Source: CAD feature listing. Evaluate the final solid. Frame: model axes, mm. A direction names the side the tool comes from. Round coordinates to 2 decimals unless told otherwise and drop trailing zeros. Order: outer loops, then holes, each group sorted by start corner. A loop starts at its lowest first (then second) coordinate and runs counter-clockwise, first axis right, second up. Notation, with made-up numbers: (47.5, 72.5) - (103.5, 72.5) arc R28 cw to (103.5, 91.5) - close; hole circle Ø6 at (17.25, 21). An arc over 180 degrees is marked (long way). Return JSON: item names as keys, results as strings. Group by question number.
1) Section A-A, the plane y = -49. Return loops of the section in (x, z).
2) Access query for faces 4 (the conical face through (103.076, -149.812, 9.872)), 5 (the cylindrical face through (-51.524, 147.436, 4.437)), 6 (the cylindrical face through (-113.24, -66.68, 9.26)), 7 (the cylindrical face through (1.3, 155.49, 13.14)), 8 (the cylindrical face through (-56.99, -77.15, 9.86)). Directions: +Z, -Z, +X, -X, +Y, -Y. A direction counts if a zero-diameter tool reaches every point of the face in a straight line with its end or side. Return the directions, or none.
3) Mould query, pull axis X, two halves, no side actions, for faces 1 (the conical face through (-107.812, -70.585, 9.923)), 2 (the flat face through (117.5, -2, 5)), 3 (the conical face through (-101.924, 149.812, 9.872)). Classes: pulls with the +X half, pulls with the -X half, needs draft (parallel to the pull), parting line crosses it, or undercut.
4) Contact query for flat-ended pins moving along their axis: P1, Ø6, axis at y = 145, z = 10, coming from the +X side; P2, Ø5.5, axis at y = -70, z = 10, coming from the -X side; P3, Ø6.5, axis at x = 52.5, y = -140, coming from the -Z side; P4, Ø18, axis at x = -97.5, y = 140, coming from the -Z side. Output: stop coordinate, or through.
5) Ray query, line 1 (Y direction, x = 0, z = 3.5); line 2 (X direction, y = 156, z = 10); line 3 (Y direction, x = -25.5, z = 14.5). Return the intervals inside material, ascending. Write a range as from..to.
```python
from build123d import *

# Parameters (mm, degrees)
SKETCH1_W                                            = 235
SKETCH1_H                                            = 320
BOSS_EXTRUDE1_DEPTH                                  = 20
SKETCH2_W                                            = 120
SKETCH2_H                                            = 160
CUT_EXTRUDE1_DEPTH                                   = 200.515037027
FILLET1_R                                            = 10
M3_TAPPED_HOLE1_D                                    = 2.5
M3_TAPPED_HOLE1_DEPTH                                = 10
M3_TAPPED_HOLE1_CSINK_D                              = 3.05
M3_TAPPED_HOLE1_CSINK_ANGLE                          = 90
M3_TAPPED_HOLE1_TIP                                  = 0.751075774
M3_TAPPED_HOLE2_D                                    = 2.5
M3_TAPPED_HOLE2_DEPTH                                = 8
M3_TAPPED_HOLE2_CSINK_D                              = 3.05
M3_TAPPED_HOLE2_CSINK_ANGLE                          = 90
M3_TAPPED_HOLE2_TIP                                  = 0.751075774
CBORE_FOR_M8_HEXAGON_SOCKET_HEAD_CAP_SCR_D           = 8.4
CBORE_FOR_M8_HEXAGON_SOCKET_HEAD_CAP_SCR_CBORE_D     = 15
CBORE_FOR_M8_HEXAGON_SOCKET_HEAD_CAP_SCR_CBORE_DEPTH = 9
CBORE_FOR_M12_HEXAGON_SOCKET_HEAD_CAP_SC_D           = 13
CBORE_FOR_M12_HEXAGON_SOCKET_HEAD_CAP_SC_CBORE_D     = 20
CBORE_FOR_M12_HEXAGON_SOCKET_HEAD_CAP_SC_CBORE_DEPTH = 13
M8_TAPPED_HOLE1_AT_2_COUNT                           = 2
M8_TAPPED_HOLE1_AT_2_PITCH                           = 102.5
M8_TAPPED_HOLE1_AT_3_COUNT                           = 2
M8_TAPPED_HOLE1_AT_3_PITCH                           = 205
M8_TAPPED_HOLE1_AT_4_COUNT                           = 2
M8_TAPPED_HOLE1_AT_4_PITCH                           = 50
M8_TAPPED_HOLE1_AT_5_COUNT                           = 2
M8_TAPPED_HOLE1_AT_5_PITCH                           = 155
CHAMFER1_SIZE                                        = 2
M8_TAPPED_HOLE2_AT_2_COUNT                           = 2
M8_TAPPED_HOLE2_AT_2_PITCH                           = 59.289517351
M8_TAPPED_HOLE2_AT_3_COUNT                           = 2
M8_TAPPED_HOLE2_AT_3_PITCH                           = 145
M8_TAPPED_HOLE2_AT_4_COUNT                           = 2
M8_TAPPED_HOLE2_AT_4_PITCH                           = 215
M8_TAPPED_HOLE2_AT_5_COUNT                           = 2
M8_TAPPED_HOLE2_AT_5_PITCH                           = 290


with BuildPart() as part:
    # Sketch1 → Boss-Extrude1 (new body)
    with BuildSketch(Plane.XY):
        Rectangle(SKETCH1_W, SKETCH1_H)
    extrude(amount=BOSS_EXTRUDE1_DEPTH)

    # Sketch2 → Cut-Extrude1 (cut, through all)
    with BuildSketch(Plane.XY.offset(20)):
        Rectangle(SKETCH2_W, SKETCH2_H)
    extrude(amount=-CUT_EXTRUDE1_DEPTH, mode=Mode.SUBTRACT)

    # Fillet1
    fillet1_edges = [part.edges().sort_by_distance(p)[0] for p in [
        (60, 80, 10),
        (60, -80, 10),
        (-60, -80, 10),
        (-60, 80, 10),
    ]]
    fillet(fillet1_edges, radius=FILLET1_R)

    # M3 Tapped Hole1
    with Locations(Plane(origin=(0, 0, 0), x_dir=(-1, 0, 0), z_dir=(0, 0, -1))):
        with Locations((-95, 65), (-105, 0), (-95, -65), (-65, 145), (0, 155), (65, 145)):
            CounterSinkHole(M3_TAPPED_HOLE1_D / 2, M3_TAPPED_HOLE1_CSINK_D / 2, depth=M3_TAPPED_HOLE1_DEPTH, counter_sink_angle=M3_TAPPED_HOLE1_CSINK_ANGLE)
            with Locations((0, 0, -(M3_TAPPED_HOLE1_DEPTH + M3_TAPPED_HOLE1_TIP / 2))):  # 118° drill point
                Cone(0, M3_TAPPED_HOLE1_D / 2, M3_TAPPED_HOLE1_TIP, mode=Mode.SUBTRACT)

    # M3 Tapped Hole2
    with Locations(Plane(origin=(0, 0, 0), x_dir=(-1, 0, 0), z_dir=(0, 0, -1))):
        with Locations((110, -105), (80, -140), (65, -140), (110, -120)):
            CounterSinkHole(M3_TAPPED_HOLE2_D / 2, M3_TAPPED_HOLE2_CSINK_D / 2, depth=M3_TAPPED_HOLE2_DEPTH, counter_sink_angle=M3_TAPPED_HOLE2_CSINK_ANGLE)
            with Locations((0, 0, -(M3_TAPPED_HOLE2_DEPTH + M3_TAPPED_HOLE2_TIP / 2))):  # 118° drill point
                Cone(0, M3_TAPPED_HOLE2_D / 2, M3_TAPPED_HOLE2_TIP, mode=Mode.SUBTRACT)

    # CBORE for M8 Hexagon socket head cap screws1 (through all)
    with Locations(Plane(origin=(0, 0, 0), x_dir=(-1, 0, 0), z_dir=(0, 0, -1))):
        with Locations((-52.5, 140), (-97.5, 95), (52.5, 140), (97.5, 95), (-97.5, -95), (-52.5, -140), (52.5, -140), (97.5, -95)):
            CounterBoreHole(CBORE_FOR_M8_HEXAGON_SOCKET_HEAD_CAP_SCR_D / 2, CBORE_FOR_M8_HEXAGON_SOCKET_HEAD_CAP_SCR_CBORE_D / 2, CBORE_FOR_M8_HEXAGON_SOCKET_HEAD_CAP_SCR_CBORE_DEPTH)

    # CBORE for M12 Hexagon socket head cap screws2 (through all)
    with Locations(Plane(origin=(0, 0, 0), x_dir=(-1, 0, 0), z_dir=(0, 0, -1))):
        with Locations((-97.5, 140), (97.5, 140), (-97.5, -140), (97.5, -140)):
            CounterBoreHole(CBORE_FOR_M12_HEXAGON_SOCKET_HEAD_CAP_SC_D / 2, CBORE_FOR_M12_HEXAGON_SOCKET_HEAD_CAP_SC_CBORE_D / 2, CBORE_FOR_M12_HEXAGON_SOCKET_HEAD_CAP_SC_CBORE_DEPTH)

    # Sketch24 → M8 Tapped Hole1 (revolve, cut)
    with BuildSketch(Plane(origin=(-102.5, 160, 10), x_dir=(0, 0, 1), z_dir=(1, 0, 0))):
        Polygon((0, 0), (0, 10.542926105), (3.4, 8.5), (3.4, 0.625), (4.025, 0), align=None)
    m8_tapped_hole1 = revolve(axis=Axis((-102.5, 166.35, 10), (0, -1, 0)), mode=Mode.SUBTRACT)

    # M8 Tapped Hole1 at 2: M8 Tapped Hole1 ×2
    with Locations(*[(i * M8_TAPPED_HOLE1_AT_2_PITCH, 0, 0) for i in range(1, M8_TAPPED_HOLE1_AT_2_COUNT)]):
        add(m8_tapped_hole1, mode=Mode.SUBTRACT)

    # M8 Tapped Hole1 at 3: M8 Tapped Hole1 ×2
    with Locations(*[(i * M8_TAPPED_HOLE1_AT_3_PITCH, 0, 0) for i in range(1, M8_TAPPED_HOLE1_AT_3_COUNT)]):
        add(m8_tapped_hole1, mode=Mode.SUBTRACT)

    # M8 Tapped Hole1 at 4: M8 Tapped Hole1 ×2
    with Locations(*[(i * M8_TAPPED_HOLE1_AT_4_PITCH, 0, 0) for i in range(1, M8_TAPPED_HOLE1_AT_4_COUNT)]):
        add(m8_tapped_hole1, mode=Mode.SUBTRACT)

    # M8 Tapped Hole1 at 5: M8 Tapped Hole1 ×2
    with Locations(*[(i * M8_TAPPED_HOLE1_AT_5_PITCH, 0, 0) for i in range(1, M8_TAPPED_HOLE1_AT_5_COUNT)]):
        add(m8_tapped_hole1, mode=Mode.SUBTRACT)

    # Mirror1: M8 Tapped Hole1 across plane
    add(m8_tapped_hole1.mirror(Plane.ZX), mode=Mode.SUBTRACT)

    # Mirror1 copy 1 sketch → Mirror1 copy 1 (revolve, cut)
    with BuildSketch(Plane(origin=(0, -160, 10), x_dir=(0, 0, 1), z_dir=(1, 0, 0))):
        Polygon((0, 0), (0, -10.542926105), (3.4, -8.5), (3.4, -0.625), (4.025, 0), align=None)
    revolve(axis=Axis((0, -166.35, 10), (0, -1, 0)), mode=Mode.SUBTRACT)

    # Mirror1 copy 2 sketch → Mirror1 copy 2 (revolve, cut)
    with BuildSketch(Plane(origin=(102.5, -160, 10), x_dir=(0, 0, 1), z_dir=(1, 0, 0))):
        Polygon((0, 0), (0, -10.542926105), (3.4, -8.5), (3.4, -0.625), (4.025, 0), align=None)
    revolve(axis=Axis((102.5, -166.35, 10), (0, -1, 0)), mode=Mode.SUBTRACT)

    # Mirror1 copy 3 sketch → Mirror1 copy 3 (revolve, cut)
    with BuildSketch(Plane(origin=(-52.5, -160, 10), x_dir=(0, 0, 1), z_dir=(1, 0, 0))):
        Polygon((0, 0), (0, -10.542926105), (3.4, -8.5), (3.4, -0.625), (4.025, 0), align=None)
    revolve(axis=Axis((-52.5, -166.35, 10), (0, -1, 0)), mode=Mode.SUBTRACT)

    # Mirror1 copy 4 sketch → Mirror1 copy 4 (revolve, cut)
    with BuildSketch(Plane(origin=(52.5, -160, 10), x_dir=(0, 0, 1), z_dir=(1, 0, 0))):
        Polygon((0, 0), (0, -10.542926105), (3.4, -8.5), (3.4, -0.625), (4.025, 0), align=None)
    revolve(axis=Axis((52.5, -166.35, 10), (0, -1, 0)), mode=Mode.SUBTRACT)

    # Chamfer1
    chamfer1_edges = [part.edges().sort_by_distance(p)[0] for p in [
        (117.5, -160, 10),
        (-117.5, -160, 10),
        (-117.5, 160, 10),
        (117.5, 160, 10),
    ]]
    chamfer(chamfer1_edges, length=CHAMFER1_SIZE)

    # Sketch27 → M8 Tapped Hole2 (revolve, cut)
    with BuildSketch(Plane(origin=(-117.5, 145, 10), x_dir=(0, 0, 1), z_dir=(0, 1, 0))):
        Polygon((0, 0), (0, 10.042926105), (3.4, 8), (3.4, 0.625), (4.025, 0), align=None)
    m8_tapped_hole2 = revolve(axis=Axis((-123.85, 145, 10), (1, 0, 0)), mode=Mode.SUBTRACT)

    # M8 Tapped Hole2 at 2: M8 Tapped Hole2 ×2
    with Locations(*[(0, -i * M8_TAPPED_HOLE2_AT_2_PITCH, 0) for i in range(1, M8_TAPPED_HOLE2_AT_2_COUNT)]):
        add(m8_tapped_hole2, mode=Mode.SUBTRACT)

    # M8 Tapped Hole2 at 3: M8 Tapped Hole2 ×2
    with Locations(*[(0, -i * M8_TAPPED_HOLE2_AT_3_PITCH, 0) for i in range(1, M8_TAPPED_HOLE2_AT_3_COUNT)]):
        add(m8_tapped_hole2, mode=Mode.SUBTRACT)

    # M8 Tapped Hole2 at 4: M8 Tapped Hole2 ×2
    with Locations(*[(0, -i * M8_TAPPED_HOLE2_AT_4_PITCH, 0) for i in range(1, M8_TAPPED_HOLE2_AT_4_COUNT)]):
        add(m8_tapped_hole2, mode=Mode.SUBTRACT)

    # M8 Tapped Hole2 at 5: M8 Tapped Hole2 ×2
    with Locations(*[(0, -i * M8_TAPPED_HOLE2_AT_5_PITCH, 0) for i in range(1, M8_TAPPED_HOLE2_AT_5_COUNT)]):
        add(m8_tapped_hole2, mode=Mode.SUBTRACT)

    # Mirror2: M8 Tapped Hole2 across plane
    add(m8_tapped_hole2.mirror(Plane(origin=(0, 0, 0), x_dir=(0, 0, 1), z_dir=(1, 0, 0))), mode=Mode.SUBTRACT)

    # Mirror2 copy 1 sketch → Mirror2 copy 1 (revolve, cut)
    with BuildSketch(Plane(origin=(117.5, 85.710482649, 10), x_dir=(0, 0, 1), z_dir=(0, 1, 0))):
        Polygon((0, 0), (0, -10.042926105), (3.4, -8), (3.4, -0.625), (4.025, 0), align=None)
    revolve(axis=Axis((123.85, 85.710482649, 10), (1, 0, 0)), mode=Mode.SUBTRACT)

    # Mirror2 copy 2 sketch → Mirror2 copy 2 (revolve, cut)
    with BuildSketch(Plane(origin=(117.5, 0, 10), x_dir=(0, 0, 1), z_dir=(0, 1, 0))):
        Polygon((0, 0), (0, -10.042926105), (3.4, -8), (3.4, -0.625), (4.025, 0), align=None)
    revolve(axis=Axis((123.85, 0, 10), (1, 0, 0)), mode=Mode.SUBTRACT)

    # Mirror2 copy 3 sketch → Mirror2 copy 3 (revolve, cut)
    with BuildSketch(Plane(origin=(117.5, -70, 10), x_dir=(0, 0, 1), z_dir=(0, 1, 0))):
        Polygon((0, 0), (0, -10.042926105), (3.4, -8), (3.4, -0.625), (4.025, 0), align=None)
    revolve(axis=Axis((123.85, -70, 10), (1, 0, 0)), mode=Mode.SUBTRACT)

    # Mirror2 copy 4 sketch → Mirror2 copy 4 (revolve, cut)
    with BuildSketch(Plane(origin=(117.5, -145, 10), x_dir=(0, 0, 1), z_dir=(0, 1, 0))):
        Polygon((0, 0), (0, -10.042926105), (3.4, -8), (3.4, -0.625), (4.025, 0), align=None)
    revolve(axis=Axis((123.85, -145, 10), (1, 0, 0)), mode=Mode.SUBTRACT)


solid = part.part
```
Geometry check:
{
 "1": {"outline": "(-117.5, 0) - (-60, 0) - (-60, 20) - (-117.5, 20) - close; (60, 0) - (117.5, 0) - (117.5, 20) - (60, 20) - close"},
 "2": {"face 4": "-Y", "face 5": "-Z", "face 6": "-X", "face 7": "+Y", "face 8": "+Z, -Z"},
 "3": {"face 1": "pulls with the -X half", "face 2": "pulls with the +X half", "face 3": "undercut"},
 "4": {"P1": "x = 109.26", "P2": "x = -109.11", "P3": "through", "P4": "z = 13"},
 "5": {"line 1": "-160..-80, 80..153.75, 156.25..160", "line 2": "-117.5..-105.9, -99.1..-55.9, -49.1..-3.4, 3.4..49.1, 55.9..99.1, 105.9..117.5", "line 3": "-160..-80, 80..160"}
}
